```python
from build123d import *

# Parameters (mm, degrees)
BOX548_W                     = 6
BOX548_H                     = 8
BOX548_DEPTH                 = 2
BOX548_PLACEMENT_ANGLE       = 45
BOX546_W                     = 6
BOX546_H                     = 8
BOX546_DEPTH                 = 2
BOX545_W                     = 6
BOX545_H                     = 8
BOX545_DEPTH                 = 2
BOX549_W                     = 6
BOX549_H                     = 8
BOX549_DEPTH                 = 2
BOX549_PLACEMENT_ANGLE       = 135
BOX550_W                     = 6
BOX550_H                     = 8
BOX550_DEPTH                 = 2
BOX547_W                     = 6
BOX547_H                     = 8
BOX547_DEPTH                 = 2
BOX547_PLACEMENT_ANGLE       = 225
BOX551_W                     = 6
BOX551_H                     = 8
BOX551_DEPTH                 = 2
BOX544_W                     = 6
BOX544_H                     = 8
BOX544_DEPTH                 = 2
BOX544_PLACEMENT_ANGLE       = 45
COMPOUND925_PLACEMENT_ANGLE  = 22.5
CYLINDER1290_R               = 1.5
CYLINDER1290_DEPTH           = 32
CYLINDER1290_PLACEMENT_ANGLE = 45
CYLINDER1293_R               = 1.5
CYLINDER1293_DEPTH           = 32
CYLINDER1291_R               = 1.5
CYLINDER1291_DEPTH           = 32
CYLINDER1291_PLACEMENT_ANGLE = 135
CYLINDER1289_R               = 1.5
CYLINDER1289_DEPTH           = 32
CYLINDER1287_R               = 1.5
CYLINDER1287_DEPTH           = 32
CYLINDER1287_PLACEMENT_ANGLE = 225
CYLINDER1292_R               = 1.5
CYLINDER1292_DEPTH           = 32
CYLINDER1286_R               = 1.5
CYLINDER1286_DEPTH           = 32
CYLINDER1286_PLACEMENT_ANGLE = 45
CYLINDER1288_R               = 1.5
CYLINDER1288_DEPTH           = 32
COMPOUND926_PLACEMENT_ANGLE  = 22.5
TUBE115_R                    = 50
TUBE115_R_2                  = 40
TUBE115_DEPTH                = 12
TUBE113_R                    = 46
TUBE113_R_2                  = 40
TUBE113_DEPTH                = 24


with BuildPart() as krychle548:
    # Box548 → Box548 (new body)
    with BuildSketch(Plane.XY):
        with Locations((3, 4)):
            Rectangle(BOX548_W, BOX548_H)
    extrude(amount=BOX548_DEPTH)


with BuildPart() as krychle548_1:
    # Box548 placement: moved
    add(krychle548.part.moved(Location((30.405592, -34.648232, 33))).rotate(Axis((30.405592, -34.648232, 33), (0, 0, 1)), BOX548_PLACEMENT_ANGLE))


with BuildPart() as krychle546:
    # Box546 → Box546 (new body)
    with BuildSketch(Plane(origin=(46, -3, 33), x_dir=(0, 1, 0), z_dir=(0, 0, 1))):
        with Locations((3, 4)):
            Rectangle(BOX546_W, BOX546_H)
    extrude(amount=BOX546_DEPTH)


with BuildPart() as krychle545:
    # Box545 → Box545 (new body)
    with BuildSketch(Plane(origin=(-3, -46, 33), x_dir=(1, 0, 0), z_dir=(0, 0, 1))):
        with Locations((3, 4)):
            Rectangle(BOX545_W, BOX545_H)
    extrude(amount=BOX545_DEPTH)


with BuildPart() as krychle549:
    # Box549 → Box549 (new body)
    with BuildSketch(Plane.XY):
        with Locations((3, 4)):
            Rectangle(BOX549_W, BOX549_H)
    extrude(amount=BOX549_DEPTH)


with BuildPart() as krychle549_1:
    # Box549 placement: moved
    add(krychle549.part.moved(Location((34.648232, 30.405592, 33))).rotate(Axis((34.648232, 30.405592, 33), (0, 0, 1)), BOX549_PLACEMENT_ANGLE))


with BuildPart() as krychle550:
    # Box550 → Box550 (new body)
    with BuildSketch(Plane(origin=(3, 46, 33), x_dir=(-1, 0, 0), z_dir=(0, 0, 1))):
        with Locations((3, 4)):
            Rectangle(BOX550_W, BOX550_H)
    extrude(amount=BOX550_DEPTH)


with BuildPart() as krychle547:
    # Box547 → Box547 (new body)
    with BuildSketch(Plane.XY):
        with Locations((3, 4)):
            Rectangle(BOX547_W, BOX547_H)
    extrude(amount=BOX547_DEPTH)


with BuildPart() as krychle547_1:
    # Box547 placement: moved
    add(krychle547.part.moved(Location((-30.405592, 34.648232, 33))).rotate(Axis((-30.405592, 34.648232, 33), (0, 0, 1)), BOX547_PLACEMENT_ANGLE))


with BuildPart() as krychle551:
    # Box551 → Box551 (new body)
    with BuildSketch(Plane(origin=(-46, 3, 33), x_dir=(0, -1, 0), z_dir=(0, 0, 1))):
        with Locations((3, 4)):
            Rectangle(BOX551_W, BOX551_H)
    extrude(amount=BOX551_DEPTH)


with BuildPart() as compound925:
    # Box544 → Box544 (new body)
    with BuildSketch(Plane.XY):
        with Locations((3, 4)):
            Rectangle(BOX544_W, BOX544_H)
    extrude(amount=BOX544_DEPTH)


with BuildPart() as compound925_1:
    # Box544 placement: moved
    add(compound925.part.moved(Location((-34.648232, -30.405592, 33))).rotate(Axis((-34.648232, -30.405592, 33), (0, 0, -1)), BOX544_PLACEMENT_ANGLE))

    # Compound925: union Krychle548, Krychle546, Krychle545, Krychle549, Krychle550, Krychle547, Krychle551
    add(krychle548_1.part)
    add(krychle546.part)
    add(krychle545.part)
    add(krychle549_1.part)
    add(krychle550.part)
    add(krychle547_1.part)
    add(krychle551.part)


with BuildPart() as compound925_2:
    # Compound925 placement: moved
    add(compound925_1.part.moved(Location((0, 0, 10))).rotate(Axis((0, 0, 10), (0, 0, 1)), COMPOUND925_PLACEMENT_ANGLE))


with BuildPart() as obj1:
    # Cylinder1290 → Cylinder1290 (new body)
    with BuildSketch(Plane.XY):
        Circle(CYLINDER1290_R)
    extrude(amount=CYLINDER1290_DEPTH)


with BuildPart() as obj1_1:
    # Cylinder1290 placement: moved
    add(obj1.part.moved(Location((29.698485, -29.698485, 33.5))).rotate(Axis((29.698485, -29.698485, 33.5), (0, 0, 1)), CYLINDER1290_PLACEMENT_ANGLE))


with BuildPart() as obj2:
    # Cylinder1293 → Cylinder1293 (new body)
    with BuildSketch(Plane(origin=(42, 0, 33.5), x_dir=(0, 1, 0), z_dir=(0, 0, 1))):
        Circle(CYLINDER1293_R)
    extrude(amount=CYLINDER1293_DEPTH)


with BuildPart() as obj3:
    # Cylinder1291 → Cylinder1291 (new body)
    with BuildSketch(Plane.XY):
        Circle(CYLINDER1291_R)
    extrude(amount=CYLINDER1291_DEPTH)


with BuildPart() as obj3_1:
    # Cylinder1291 placement: moved
    add(obj3.part.moved(Location((29.698485, 29.698485, 33.5))).rotate(Axis((29.698485, 29.698485, 33.5), (0, 0, 1)), CYLINDER1291_PLACEMENT_ANGLE))


with BuildPart() as obj4:
    # Cylinder1289 → Cylinder1289 (new body)
    with BuildSketch(Plane(origin=(0, 42, 33.5), x_dir=(-1, 0, 0), z_dir=(0, 0, 1))):
        Circle(CYLINDER1289_R)
    extrude(amount=CYLINDER1289_DEPTH)


with BuildPart() as obj5:
    # Cylinder1287 → Cylinder1287 (new body)
    with BuildSketch(Plane.XY):
        Circle(CYLINDER1287_R)
    extrude(amount=CYLINDER1287_DEPTH)


with BuildPart() as obj5_1:
    # Cylinder1287 placement: moved
    add(obj5.part.moved(Location((-29.698485, 29.698485, 33.5))).rotate(Axis((-29.698485, 29.698485, 33.5), (0, 0, 1)), CYLINDER1287_PLACEMENT_ANGLE))


with BuildPart() as obj6:
    # Cylinder1292 → Cylinder1292 (new body)
    with BuildSketch(Plane(origin=(-42, 0, 33.5), x_dir=(0, -1, 0), z_dir=(0, 0, 1))):
        Circle(CYLINDER1292_R)
    extrude(amount=CYLINDER1292_DEPTH)


with BuildPart() as obj7:
    # Cylinder1286 → Cylinder1286 (new body)
    with BuildSketch(Plane.XY):
        Circle(CYLINDER1286_R)
    extrude(amount=CYLINDER1286_DEPTH)


with BuildPart() as obj7_1:
    # Cylinder1286 placement: moved
    add(obj7.part.moved(Location((-29.698485, -29.698485, 33.5))).rotate(Axis((-29.698485, -29.698485, 33.5), (0, 0, -1)), CYLINDER1286_PLACEMENT_ANGLE))


with BuildPart() as compound926:
    # Cylinder1288 → Cylinder1288 (new body)
    with BuildSketch(Plane(origin=(0, -42, 33.5), x_dir=(1, 0, 0), z_dir=(0, 0, 1))):
        Circle(CYLINDER1288_R)
    extrude(amount=CYLINDER1288_DEPTH)

    # Compound926: union obj1, obj2, obj3, obj4, obj5, obj6, obj7
    add(obj1_1.part)
    add(obj2.part)
    add(obj3_1.part)
    add(obj4.part)
    add(obj5_1.part)
    add(obj6.part)
    add(obj7_1.part)


with BuildPart() as compound926_1:
    # Compound926 placement: moved
    add(compound926.part.moved(Location((0, 0, 3))).rotate(Axis((0, 0, 3), (0, 0, 1)), COMPOUND926_PLACEMENT_ANGLE))


with BuildPart() as tube115:
    # Tube115 → Tube115 (new body)
    with BuildSketch(Plane.XY.offset(24)):
        Circle(TUBE115_R)
        Circle(TUBE115_R_2, mode=Mode.SUBTRACT)
    extrude(amount=TUBE115_DEPTH)


with BuildPart() as cut476:
    # Tube113 → Tube113 (new body)
    with BuildSketch(Plane.XY.offset(25)):
        Circle(TUBE113_R)
        Circle(TUBE113_R_2, mode=Mode.SUBTRACT)
    extrude(amount=TUBE113_DEPTH)

    # Cut473: cut Tube115
    add(tube115.part, mode=Mode.SUBTRACT)

    # Cut475: cut Compound926
    add(compound926_1.part, mode=Mode.SUBTRACT)

    # Cut476: cut Compound925
    add(compound925_2.part, mode=Mode.SUBTRACT)


solid = cut476.part
```
Could you check a few things on this model? Use its own coordinates, in mm. A direction names the side the tool comes from. Coordinates: 2 decimals unless noted, no trailing zeros. Write each loop counter-clockwise with the first axis right and the second up, starting at its lowest first coordinate (ties: lowest second). Pieces come first, ordered by that corner, then holes. Notation, with made-up numbers: (82, -8) -> (119, -8) arc R24 cw to (119, 22) -> close; hole circle Ø7 at (10, -19). An arc over 180 degrees is marked (long way). Return JSON: item names as keys, results as strings.
(1) We'd pull the mould along X, two halves only. Please class faces 3 (the cylindrical face through (-33.904, 31.089, 42.409)), 4 (the flat face through (-16, -41, 45)): +X half, -X half, draft (parallel to the pull), parting line (faces both ways), or undercut.
Numbers:
{"face 3": "parting line", "face 4": "undercut"}
(2) Imagine slicing it at A-A, the plane y = 0. Please give me the cut outline in (x, z), then the cut area to 3 significant figures.
Numbers:
{"outline": "(-46, 36) -> (-40, 36) -> (-40, 49) -> (-46, 49) -> close; (40, 36) -> (46, 36) -> (46, 49) -> (40, 49) -> close", "area": "156 mm2"}
(3) Which directions (+Z, -Z, +X, -X, +Y, -Y) give clear straight access to the entire face, cutting with the end or side of a thin tool? Please do faces 1 (the flat face through (-13.66, 40.82, 43.99)), 2 (the cylindrical face through (-37.943, 14.844, 46.972)).
Numbers:
{"face 1": "none", "face 2": "+Z"}
(4) Imagine slicing it at C-C, the plane z = 40.25. Count the separate pieces of the cut face and the enclosed holes in it, then the cut area to 3 significant figures.
Numbers:
{"separate pieces": "1", "enclosed holes": "9", "area": "1,560 mm2"}
(5) I'm going to push flat-ended pins straight in: pin 1 (5 mm diameter, centred on x = -11.5, z = 40.5, fed in from +Y); pin 2 (6 mm diameter, centred on x = 10, z = 42, fed in from -Y); pin 3 (2.5 mm diameter, centred on x = -38.8, y = 16.07, fed in from +Z). Where does each tip first touch, or does it pass through?
Numbers:
{"pin 1": "stops at y = 45.11", "pin 2": "stops at y = -45.46", "pin 3": "stops at z = 36.5"}
(6) I need wall thicknesses on L1, parallel to Z at x = -14.5, y = -40.5; L2, parallel to Y at x = -16.5, z = 45.5; L3, parallel to Y at x = 40.5, z = 43.75. Which ranges of each line are inside material? Lowest first, please.
Numbers:
{"L1": "z = 36 to 43, 45 to 49", "L2": "y = -42.94 to -40.24, -37.37 to -36.44, 36.44 to 37.37, 40.24 to 42.94", "L3": "y = -21.81 to -20.02, -13.53 to 13.53, 20.02 to 21.81"}
